```python
from build123d import *

# Parameters (mm, degrees)
SKETCH1_R           = 20
BOSS_EXTRUDE1_DEPTH = 3
CUT_EXTRUDE2_DEPTH  = 3
SKETCH4_R           = 2.125
CUT_EXTRUDE3_DEPTH  = 10


with BuildPart() as part:
    # Sketch1 → Boss-Extrude1 (new body)
    with BuildSketch(Plane.XY):
        Circle(SKETCH1_R)
    extrude(amount=BOSS_EXTRUDE1_DEPTH)

    # Sketch3 → Cut-Extrude2 (cut)
    with BuildSketch(Plane.XY.offset(3)):
        Polygon((0, 4.041451884), (-3.5, 2.020725942), (-3.5, -2.020725942), (0, -4.041451884), (3.5, -2.020725942), (3.5, 2.020725942), align=None)
    extrude(amount=-CUT_EXTRUDE2_DEPTH, mode=Mode.SUBTRACT)

    # Sketch4 → Cut-Extrude3 (cut)
    with BuildSketch(Plane.XY.offset(3)):
        with Locations((0, 12)):
            Circle(SKETCH4_R)
        with Locations((12, 0)):
            Circle(SKETCH4_R)
        with Locations((0, -12)):
            Circle(SKETCH4_R)
        with Locations((-12, 0)):
            Circle(SKETCH4_R)
    extrude(amount=-CUT_EXTRUDE3_DEPTH, mode=Mode.SUBTRACT)


solid = part.part
```
Geometry: final body of the model. Coordinates: model frame, mm. A direction names the side the tool comes from. Round coordinates to 2 decimals unless told otherwise and drop trailing zeros. Write each loop counter-clockwise with the first axis right and the second up, starting at its lowest first coordinate (ties: lowest second). Pieces come first, ordered by that corner, then holes.
Item 1: Section query A-A (y = -12). Return loops of the section in (x, z) (3 decimals).
Item 2: Section query D-D (x = -16). Return loops of the section in (y, z).
Item 3: Section query C-C (z = 1.1). Return loops of the section in (x, y) (3 decimals).
Item 4: Material intervals for L1, parallel to Y at x = 0, z = 2.15 (3 decimals); L2, parallel to Y at x = -1.5, z = 2.85; L3, parallel to Y at x = 13, z = 0.7 (3 decimals), sorted ascending.
Item 5: Set-up query: faces 1 (the face through (-0.3, -4.2, 3)), 2 (the face through (1.726, -3.045, 1.521)). Return all of +Z, -Z, +X, -X, +Y, -Y with unobstructed straight access to the full face (end or side cutting, diameter ignored); none if empty.
Item 6: Mould query, pull axis Y, two halves, no side actions, for faces 3 (the face through (-4.336, -19.524, 1.479)), 4 (the face through (1.142, 13.792, 1.521)), 5 (the face through (-0.3, -4.2, 0)). Classes: +Y half, -Y half, draft (parallel to the pull), parting line (faces both ways), or undercut.
Completed:
1. outline: (-16, 0) - (-2.125, 0) - (-2.125, 3) - (-16, 3) - close; (2.125, 0) - (16, 0) - (16, 3) - (2.125, 3) - close
2. outline: (-12, 0) - (12, 0) - (12, 3) - (-12, 3) - close
3. outline: circle Ø40 at (0, 0); hole circle Ø4.25 at (-12, 0); hole (-3.5, -2.021) - (0, -4.041) - (3.5, -2.021) - (3.5, 2.021) - (0, 4.041) - (-3.5, 2.021) - close; hole circle Ø4.25 at (0, -12); hole circle Ø4.25 at (0, 12); hole circle Ø4.25 at (12, 0)
4. L1: y = -20 to -14.125, -9.875 to -4.041, 4.041 to 9.875, 14.125 to 20
4. L2: y = -19.94 to -13.51, -10.49 to -3.18, 3.18 to 10.49, 13.51 to 19.94
4. L3: y = -15.199 to -1.875, 1.875 to 15.199
5. face 1: +Z, +X, -X, +Y, -Y
5. face 2: +Z, -Z
6. face 3: parting line
6. face 4: undercut
6. face 5: draft
